from build123d import *

# Parameters (mm, degrees)
SKETCH1_W             = 5.08
SKETCH1_H             = 2.4
EXTRUDE_223_DEPTH     = 4.3
SKETCH2_W             = 4.6
SKETCH2_H             = 1.8
EXTRUDE_304_DEPTH     = 1
SKETCH3_W             = 5.08
SKETCH3_H             = 2.4
EXTRUDE_441_DEPTH     = 0.8
SKETCH4_W             = 3.8
SKETCH4_H             = 1.3
CUT_EXTRUDE_523_DEPTH = 3.7
SKETCH5_W             = 3.4
SKETCH5_H             = 0.9
CUT_EXTRUDE_605_DEPTH = 5
CUT_EXTRUDE_729_DEPTH = 3


with BuildPart() as part:
    # Sketch1 → Extrude 223 (new body)
    with BuildSketch(Plane.XY):
        Rectangle(SKETCH1_W, SKETCH1_H)
    extrude(amount=EXTRUDE_223_DEPTH)

    # Sketch2 → Extrude 304 (add)
    with BuildSketch(Plane.XY.offset(4.3)):
        Rectangle(SKETCH2_W, SKETCH2_H)
    extrude(amount=EXTRUDE_304_DEPTH)

    # Sketch3 → Extrude 441 (add)
    with BuildSketch(Plane.XY.offset(5.3)):
        Rectangle(SKETCH3_W, SKETCH3_H)
    extrude(amount=EXTRUDE_441_DEPTH)

    # Sketch4 → Cut-Extrude 523 (cut)
    with BuildSketch(Plane(origin=(0, 0, 0), x_dir=(-1, 0, 0), z_dir=(0, 0, -1))):
        Rectangle(SKETCH4_W, SKETCH4_H)
    extrude(amount=-CUT_EXTRUDE_523_DEPTH, mode=Mode.SUBTRACT)

    # Sketch5 → Cut-Extrude 605 (cut)
    with BuildSketch(Plane(origin=(0, 0, 3.7), x_dir=(-1, 0, 0), z_dir=(0, 0, -1))):
        Rectangle(SKETCH5_W, SKETCH5_H)
    extrude(amount=-CUT_EXTRUDE_605_DEPTH, mode=Mode.SUBTRACT)

    # Sketch7 → Cut-Extrude 729 (cut)
    with BuildSketch(Plane.XZ.offset(1.2)):
        with BuildLine():
            Line((-0.75, 6.1), (-0.75, 4.3))
            ThreePointArc((-0.75, 4.3), (0, 3.55), (0.75, 4.3))
            Line((0.75, 4.3), (0.75, 6.1))
            Line((0.75, 6.1), (-0.75, 6.1))
        make_face()
    extrude(amount=-CUT_EXTRUDE_729_DEPTH, mode=Mode.SUBTRACT)


solid = part.part
Verification items for the finished model (mm, model axes). A direction names the side the tool comes from. Round coordinates to 2 decimals unless told otherwise and drop trailing zeros. Loops run counter-clockwise (first coordinate to the right, second up) from the corner with the lowest first, then second, coordinate; pieces in that order, holes last. Notation, with made-up numbers: (70.5, 52) - (83.5, 52) arc R16 cw to (83.5, 78) - close; hole circle Ø9 at (-38.5, 15.25). An arc over 180 degrees is marked (long way). Use a Markdown table: item, result. Add a question column.
1. Section check B-B, the plane y = 0.3. Record the boundary of the cut face in (x, z).
2. Release check for a two-part mould opening along Y. For faces 1 (the face through (1, 0.45, 5)), 2 (the face through (2, 0.9, 5)), 3 (the face through (0, -0.65, 2)), 4 (the face through (0, 1, 0)) record: released by +Y, released by -Y, zero draft, split by the parting line, or undercut.
3. Section check C-C, the plane x = 2.1. Record the boundary of the cut face in (y, z), plus the area to 3 significant figures.
4. Section check A-A, the plane x = 0. Record the boundary of the cut face in (y, z).
5. Access from +Z, -Z, +X, -X, +Y, -Y to the whole of each face (thin tool, end or side, straight path). Record for faces 5 (the face through (2.3, 0, 5)), 6 (the face through (-1, -0.45, 5)), 7 (the face through (-1.9, 0, 2)), 8 (the face through (-2.3, 0, 5)).
6. Section check D-D, the plane y = 0.75. Record the boundary of the cut face in (x, z).
7. Thickness scan on probe 1 along X at (y, z) = (-0.8, 4.75); probe 2 along Y at (x, z) = (-0.2, 1.5). Record the ranges inside material, lowest first. Write a range as [from, to].
Checks:
| question | item | result |
|---|---|---|
| 1 | outline | (-2.54, 0) - (-1.9, 0) - (-1.9, 3.7) - (-1.7, 3.7) - (-1.7, 6.1) - (-2.54, 6.1) - (-2.54, 5.3) - (-2.3, 5.3) - (-2.3, 4.3) - (-2.54, 4.3) - close; (1.7, 3.7) - (1.9, 3.7) - (1.9, 0) - (2.54, 0) - (2.54, 4.3) - (2.3, 4.3) - (2.3, 5.3) - (2.54, 5.3) - (2.54, 6.1) - (1.7, 6.1) - close |
| 2 | face 1 | undercut |
| 2 | face 2 | released by +Y |
| 2 | face 3 | undercut |
| 2 | face 4 | zero draft |
| 3 | outline | (-1.2, 0) - (1.2, 0) - (1.2, 4.3) - (0.9, 4.3) - (0.9, 5.3) - (1.2, 5.3) - (1.2, 6.1) - (-1.2, 6.1) - (-1.2, 5.3) - (-0.9, 5.3) - (-0.9, 4.3) - (-1.2, 4.3) - close |
| 3 | area | 14.0 mm^2 |
| 4 | outline | (-1.2, 0) - (-0.65, 0) - (-0.65, 3.55) - (-1.2, 3.55) - close; (0.65, 0) - (1.2, 0) - (1.2, 3.55) - (0.65, 3.55) - close |
| 5 | face 5 | +X, +Y, -Y |
| 5 | face 6 | +Z, -Z |
| 5 | face 7 | -Z |
| 5 | face 8 | -X, +Y, -Y |
| 6 | outline | (-2.54, 0) - (2.54, 0) - (2.54, 4.3) - (2.3, 4.3) - (2.3, 5.3) - (2.54, 5.3) - (2.54, 6.1) - (0.75, 6.1) - (0.75, 4.3) arc R0.75 cw to (-0.75, 4.3) - (-0.75, 6.1) - (-2.54, 6.1) - (-2.54, 5.3) - (-2.3, 5.3) - (-2.3, 4.3) - (-2.54, 4.3) - close |
| 7 | probe 1 | x = [-2.3, -0.75], [0.75, 2.3] |
| 7 | probe 2 | y = [-1.2, -0.65], [0.65, 1.2] |
